Geometry check sheet. Reference: the model listing, model coordinates, mm. A direction names the side the tool comes from. Give positions to 0.01 mm unless a question says otherwise; leave off trailing zeros. Order: outer loops, then holes, each group sorted by start corner. A loop starts at its lowest first (then second) coordinate and runs counter-clockwise, first axis right, second up. Notation, with made-up numbers: M 23.5,23 L 36.5,23 A17 cw 36.5,32 Z; hole C 51,32.5 d1. An arc over 180 degrees is marked long. Put each result on its own line as item: value. Start each with the question number.
Q1. Go/stop test with flat-tipped pins: pin 1 (0.7 mm diameter, centred on x = -22, y = 0.5, fed in from -Z); pin 2 (0.7 mm diameter, centred on y = 1, z = -14.5, fed in from -X); pin 3 (1.2 mm diameter, centred on x = -10, z = 25, fed in from -Y); pin 4 (2.5 mm diameter, centred on x = -10, z = -25, fed in from +Y). Record where each tip stops, or that it passes through.
Q2. Mould release check, pull along Z, two halves, no side actions. Record for faces 3 (the flat face through (-55.2, 0.7, 32.7)), 4 (the cylindrical face through (-39, 1, -25)), 5 (the flat face through (-36, 1.4, 1)): +Z half, -Z half, draft (parallel to the pull), parting line (faces both ways), or undercut.
Q3. Section check A-A on x = -10. Record the cut outline in (y, z), then the cut area to 3 significant figures.
Q4. Section check C-C on y = 0.4. State how many separate pieces and enclosed holes the cut face has, then the cut area to 3 significant figures.
Q5. Material ranges on L1, parallel to Z at x = -38, y = 0.65; L2, parallel to X at y = 0.85, z = -6; L3, parallel to X at y = 0.45, z = 25, recorded low to high.
Q6. Section check B-B on z = -2. Record the cut outline in (x, y), then the cut area to 3 significant figures.
Q7. Access from +Z, -Z, +X, -X, +Y, -Y to the whole of each face (thin tool, end or side, straight path). Record for faces 1 (the flat face through (-55.2, 0.7, -32.7)), 2 (the flat face through (-57, 1, 25)).
Autodesk Inventor part; units mm, degrees
ref_plane "YZ Plane" through (0, 0, 0) normal (1, 0, 0) x (0, 1, 0)
ref_plane "XZ Plane" through (0, 0, 0) normal (0, 1, 0) x (-1, 0, 0)
ref_plane "XY Plane" through (0, 0, 0) normal (0, 0, 1) x (1, 0, 0)
sketch "Sketch1" plane through (0, 0, 0) normal (0, 1, 0) x (-1, 0, 0)
  line L0 (0, 0) -> (0, -22.5)
  line L1 (0, 0) -> (0, 22.5)
  line L2 (5, 27.5) -> (50, 27.5)
  line L3 (5, -27.5) -> (50, -27.5)
  line L4 (50, 27.5) -> (60.6066, 38.1066)
  line L5 (50, 27.5) -> (65, 27.5) construction
  line L6 (50, -27.5) -> (60.6066, -38.1066)
  line L7 (50, -27.5) -> (65, -27.5) construction
  line L8 (95, 0) -> (95, -5)
  line L9 (95, 0) -> (95, 5)
  arc A0 (5, 27.5) -> (0, 22.5) centre (5, 22.5) ccw
  arc A1 (0, -22.5) -> (5, -27.5) centre (5, -22.5) ccw
  line L10 (60.6066, 38.1066) -> (62.6066, 38.1066)
  line L11 (60.6066, -38.1066) -> (62.6066, -38.1066)
  spline S0 degree 4 poles (62.6066, 38.1066) (69.2667, 38.1066) (82.5868, 38.1066) (95, 24.8465) (95, 11.6155) (95, 5) knots 0 0 0 0 0 0.5 1 1 1 1 1
  spline S1 degree 4 poles (95, -5) (95, -11.6155) (95, -24.8465) (82.5868, -38.1066) (69.2667, -38.1066) (62.6066, -38.1066) knots 0 0 0 0 0 0.5 1 1 1 1 1
  line L12 (52, 0) -> (52, -20)
  line L13 (52, 0) -> (52, 20)
  line L14 (52, 20) -> (62.6066, 30.6066)
  line L15 (52, -20) -> (62.6066, -30.6066)
  line L16 (52, -20) -> (67, -20) construction
  line L17 (62.6066, 30.6066) -> (65.6066, 30.6066)
  line L18 (62.6066, -30.6066) -> (65.6066, -30.6066)
  line L19 (88, 0) -> (88, -8)
  line L20 (88, 0) -> (88, 9)
  spline S2 degree 4 poles (62.6066, 30.6066) (67.2711, 30.6066) (76.6001, 30.6066) (88, 23.7035) (88, 13.9012) (88, 9) knots 0 0 0 0 0 0.5 1 1 1 1 1
  spline S3 degree 4 poles (65.6066, -30.6066) (70.1733, -30.6066) (79.3067, -30.6066) (88, -21.6601) (88, -12.5534) (88, -8) knots 0 0 0 0 0 0.5 1 1 1 1 1
  point P0 (0, -27.5)
  point P1 (0, 27.5)
  point P2 (80, 0)
  point P3 (38, -25)
  point P4 (10, -25)
  point P5 (38, 25)
  point P6 (10, 25)
  dimension "d1" = 27.5
  dimension "d2" = 27.5
  dimension "d3" = 50
  dimension "d4" = 50
  dimension "d5" = 15
  dimension "d6" = 45
  dimension "d7" = 15
  dimension "d8" = 45
  dimension "d17" = 5
  dimension "d18" = 5
  dimension "d19" = 5
  dimension "d20" = 2
  dimension "d21" = 2
  dimension "d22" = 20
  dimension "d23" = 20
  dimension "d24" = 15
  dimension "d25" = 15
  dimension "d26" = 45
  dimension "d27" = 3
  dimension "d28" = 3
  dimension "d29" = 8
  dimension "d30" = 9
extrude "Extrusion1" add sketch "Sketch1" along normal blind 1.4
hole "Hole1" at (-38, 0, -25) at (-10, 0, -25) at (-38, 0, 25) at (-10, 0, 25) direction (0, 1, 0) diameter 2 depth 2 tip angle 118
properties part number "mainpcb-01"
Results found:
1. pin 1: stops at z = -27.5
1. pin 2: stops at x = -94.55
1. pin 3: passes through
1. pin 4: stops at y = 1.4
2. face 3: +Z half
2. face 4: undercut
2. face 5: draft
3. outline: M 0,-27.5 L 1.4,-27.5 L 1.4,-26 L 0,-26 Z; M 0,-24 L 1.4,-24 L 1.4,24 L 0,24 Z; M 0,26 L 1.4,26 L 1.4,27.5 L 0,27.5 Z
3. area: 71.4 mm^2
4. separate pieces: 1
4. enclosed holes: 5
4. area: 3,780 mm^2
5. L1: z = -27.5 to -26, -24 to 24, 26 to 27.5
5. L2: x = -95 to -88, -52 to 0
5. L3: x = -90.81 to -82.3, -57 to -39, -37 to -11, -9 to -0.67
6. outline: M -95,0 L -88,0 L -88,1.4 L -95,1.4 Z; M -52,0 L 0,0 L 0,1.4 L -52,1.4 Z
6. area: 82.6 mm^2
7. face 1: -Z, +X, +Y, -Y
7. face 2: +Y, -Y
